```python
from build123d import *
from OCP.BRepFilletAPI import BRepFilletAPI_MakeChamfer

# Parameters (mm, degrees)
BOSS_EXTRUDE1_DEPTH = 37.5
CUT_EXTRUDE1_DEPTH  = 44.937455548
CHAMFER1_SIZE       = 1.4
BOSS_EXTRUDE2_DEPTH = 12
CHAMFER2_SIZE       = 4
CHAMFER2_SIZE2      = 1.8


with BuildPart() as part:
    # Sketch2 → Boss-Extrude1 (new, symmetric)
    with BuildSketch(Plane.XY):
        Polygon((-19.5, 0), (19.5, 0), (19.5, 12), (15, 12), (15, 9), (9, 9), (9, 12), (-9, 12), (-9, 9), (-15, 9), (-15, 12), (-19.5, 12), align=None)
    extrude(amount=BOSS_EXTRUDE1_DEPTH, both=True)

    # Sketch3 → Cut-Extrude1 (cut, through all)
    with BuildSketch(Plane(origin=(0, 12, 0), x_dir=(1, 0, 0), z_dir=(0, 1, 0))):
        with BuildLine():
            ThreePointArc((-3.8, -31.273518749), (0, -32.5), (3.8, -31.273518749))
            Line((3.8, -31.273518749), (3.8, -26))
            Line((3.8, -26), (-3.8, -26))
            Line((-3.8, -26), (-3.8, -31.273518749))
        make_face()
        with BuildLine():
            Line((3.8, -26), (3.8, -31.273518749))
            ThreePointArc((3.8, -31.273518749), (5.785758377, -28.962262649), (6.5, -26))
            ThreePointArc((6.5, -26), (-2.962262649, -20.214241623), (-3.8, -31.273518749))
            Line((-3.8, -31.273518749), (-3.8, -26))
            Line((-3.8, -26), (3.8, -26))
        make_face()
        with BuildLine():
            Line((-3.8, -37.5), (3.8, -37.5))
            Line((3.8, -37.5), (3.8, -31.273518749))
            ThreePointArc((3.8, -31.273518749), (0, -32.5), (-3.8, -31.273518749))
            Line((-3.8, -31.273518749), (-3.8, -37.5))
        make_face()
    extrude(amount=-CUT_EXTRUDE1_DEPTH, mode=Mode.SUBTRACT)

    # Chamfer1
    chamfer1_edges = [part.edges().sort_by_distance(p)[0] for p in [
        (-19.5, 12, 0),
        (-15, 12, 0),
        (-9, 12, 0),
        (9, 12, 0),
        (15, 12, 0),
        (19.5, 12, 0),
        (19.5, 0, 0),
        (-19.5, 0, 0),
        (3.8, 6, 37.5),
        (-3.8, 6, 37.5),
    ]]
    chamfer(chamfer1_edges, length=CHAMFER1_SIZE)

    # Sketch4 → Boss-Extrude2 (add)
    with BuildSketch(Plane(origin=(0, 12, 0), x_dir=(1, 0, 0), z_dir=(0, 1, 0))):
        with BuildLine():
            Line((-2.8, 43.977799287), (-2.8, 49))
            Line((-2.8, 49), (2.8, 49))
            Line((2.8, 49), (2.8, 43.977799287))
            ThreePointArc((2.8, 43.977799287), (4.957948164, 46.087741426), (5.75, 49))
            ThreePointArc((5.75, 49), (-2.912258574, 53.957948164), (-2.8, 43.977799287))
        make_face()
        with BuildLine():
            Line((2.8, 49), (-2.8, 49))
            Line((-2.8, 49), (-2.8, 43.977799287))
            ThreePointArc((-2.8, 43.977799287), (0, 43.25), (2.8, 43.977799287))
            Line((2.8, 43.977799287), (2.8, 49))
        make_face()
        with BuildLine():
            ThreePointArc((2.8, 43.977799287), (0, 43.25), (-2.8, 43.977799287))
            Line((-2.8, 43.977799287), (-2.8, 37.5))
            Line((-2.8, 37.5), (2.8, 37.5))
            Line((2.8, 37.5), (2.8, 43.977799287))
        make_face()
    extrude(amount=-BOSS_EXTRUDE2_DEPTH)

    # Chamfer2: one chamfer whose edges measure the first distance from different faces: ONE call of the kernel's chamfer builder (chamfer() names one face for all edges)
    chamfer2_edges_1 = [part.edges().sort_by_distance(p)[0] for p in [
        (2.8, 0, -40.738899644),
        (2.8, 12, -40.738899644),
    ]]
    chamfer2_side_1 = [part.faces().sort_by_distance(p)[0] for p in [
        (2.8, 6, -40.738899644),
    ]]
    chamfer2_edges_2 = [part.edges().sort_by_distance(p)[0] for p in [
        (0, 12, -54.75),
        (0, 0, -54.75),
    ]]
    chamfer2_side_2 = [part.faces().sort_by_distance(p)[0] for p in [
        (0, 6, -54.75),
    ]]
    chamfer2_edges_3 = [part.edges().sort_by_distance(p)[0] for p in [
        (-2.8, 12, -40.738899644),
        (-2.8, 0, -40.738899644),
    ]]
    chamfer2_side_3 = [part.faces().sort_by_distance(p)[0] for p in [
        (-2.8, 6, -40.738899644),
    ]]
    chamfer2 = BRepFilletAPI_MakeChamfer(part.part.solid().wrapped)
    for e in chamfer2_edges_1:
        chamfer2.Add(CHAMFER2_SIZE, CHAMFER2_SIZE2, e.wrapped, chamfer2_side_1[0].wrapped)  # the first distance lies on this face
    for e in chamfer2_edges_2:
        chamfer2.Add(CHAMFER2_SIZE, CHAMFER2_SIZE2, e.wrapped, chamfer2_side_2[0].wrapped)  # the first distance lies on this face
    for e in chamfer2_edges_3:
        chamfer2.Add(CHAMFER2_SIZE, CHAMFER2_SIZE2, e.wrapped, chamfer2_side_3[0].wrapped)  # the first distance lies on this face
    add(Compound.cast(chamfer2.Shape()), mode=Mode.REPLACE)


solid = part.part
```
Part model, mm, in its own coordinate system. A direction names the side the tool comes from. Round coordinates to 2 decimals unless told otherwise and drop trailing zeros. Loops run counter-clockwise (first coordinate to the right, second up) from the corner with the lowest first, then second, coordinate; pieces in that order, holes last. Notation, with made-up numbers: (-11, 67) -> (4, 67) arc R20 cw to (4, 87) -> close; hole circle Ø5 at (21.5, -40). An arc over 180 degrees is marked (long way). Use a Markdown table: item, result.
1) Probe line 1 (X direction, y = 10.5, z = 18); line 2 (Z direction, x = 4.5, y = 7.25); line 3 (X direction, y = 8.5, z = 26). List the from-to ranges inside material, lowest first. Write a range as [from, to].
The answers:
| item | result |
|---|---|
| line 1 | x = [-19.5, -15], [-9, 9], [15, 19.5] |
| line 2 | z = [-52.58, -45.42], [-37.5, 21.31], [30.69, 36.8] |
| line 3 | x = [-19.5, -6.5], [6.5, 19.5] |
2) Pull direction X, two halves, no side cores. Call faces 5 (the flat face through (-19.5, 6, 1)), 6 (the flat face through (10, 6, -37.5)), 7 (the flat face through (-3.8, 6, 34)): pulls with the +X half, pulls with the -X half, needs draft (parallel to the pull), parting line crosses it, or undercut.
The answers:
| item | result |
|---|---|
| face 5 | pulls with the -X half |
| face 6 | needs draft |
| face 7 | undercut |
3) Tool access for faces 1 (the flat face through (-15, 10, 1)), 2 (the flat face through (-2.8, 6, -41)), 3 (the flat face through (-1.9, 10, -41.4)), 4 (the flat face through (1.9, 10, -41.3)): list every direction of +Z, -Z, +X, -X, +Y, -Y with a clear straight run to the whole face (end or side of a thin tool).
The answers:
| item | result |
|---|---|
| face 1 | +Z, -Z, +Y |
| face 2 | -X, +Y, -Y |
| face 3 | -X, +Y |
| face 4 | +X, +Y |
4) Cut at D-D, the plane x = -12. List the corners of the cut face in (y, z), and give its area (3 significant figures).
The answers:
| item | result |
|---|---|
| outline | (0, -37.5) -> (9, -37.5) -> (9, 37.5) -> (0, 37.5) -> close |
| area | 675 mm2 |
5) Drop flat-ended pins along their axis: pin 1 Ø1 at (x, y) = (10.5, 3) entering from -Z; pin 2 Ø15 at (x, z) = (0, 26) entering from +Y; pin 3 Ø3 at (y, z) = (6, -39.5) entering from -X; pin 4 Ø2 at (y, z) = (6, -42.5) entering from +X. Give the stop position or say it passes through.
The answers:
| item | result |
|---|---|
| pin 1 | stops at z = -37.5 |
| pin 2 | stops at y = 12 |
| pin 3 | stops at x = -2.8 |
| pin 4 | stops at x = 2.8 |
6) Cut at B-B, the plane y = 5.75. List the corners of the cut face in (x, z), and give its area (3 significant figures).
The answers:
| item | result |
|---|---|
| outline | (-19.5, -37.5) -> (-2.8, -37.5) -> (-2.8, -43.98) arc R5.75 ccw (long way) to (2.8, -43.98) -> (2.8, -37.5) -> (19.5, -37.5) -> (19.5, 37.5) -> (5.2, 37.5) -> (3.8, 36.1) -> (3.8, 31.27) arc R6.5 cw (long way) to (-3.8, 31.27) -> (-3.8, 36.1) -> (-5.2, 37.5) -> (-19.5, 37.5) -> close |
| area | 2,890 mm2 |
7) Cut at C-C, the plane x = 0. List the corners of the cut face in (y, z), and give its area (3 significant figures).
The answers:
| item | result |
|---|---|
| outline | (0, -52.95) -> (4, -54.75) -> (8, -54.75) -> (12, -52.95) -> (12, 19.5) -> (0, 19.5) -> close |
| area | 884 mm2 |
8) Cut at A-A, the plane z = -9.5. List the corners of the cut face in (x, y).
The answers:
| item | result |
|---|---|
| outline | (-19.5, 1.4) -> (-18.1, 0) -> (18.1, 0) -> (19.5, 1.4) -> (19.5, 10.6) -> (18.1, 12) -> (16.4, 12) -> (15, 10.6) -> (15, 9) -> (9, 9) -> (9, 10.6) -> (7.6, 12) -> (-7.6, 12) -> (-9, 10.6) -> (-9, 9) -> (-15, 9) -> (-15, 10.6) -> (-16.4, 12) -> (-18.1, 12) -> (-19.5, 10.6) -> close |
